The listing builds one solid part. Answer for the finished solid, in the listing's coordinates (mm). Face numbers are marked on the shaded views. Round coordinates to 2 decimals unless told otherwise and drop trailing zeros. Write each loop counter-clockwise with the first axis right and the second up, starting at its lowest first coordinate (ties: lowest second). Pieces come first, ordered by that corner, then holes. Notation, with made-up numbers: (64, 58.5) -> (123, 58.5) arc R5 cw to (123, 65.5) -> close; hole circle Ø11 at (25, 26). An arc over 180 degrees is marked (long way). Write each question's results on one line, items separated by ' | '. Start each with the question number.
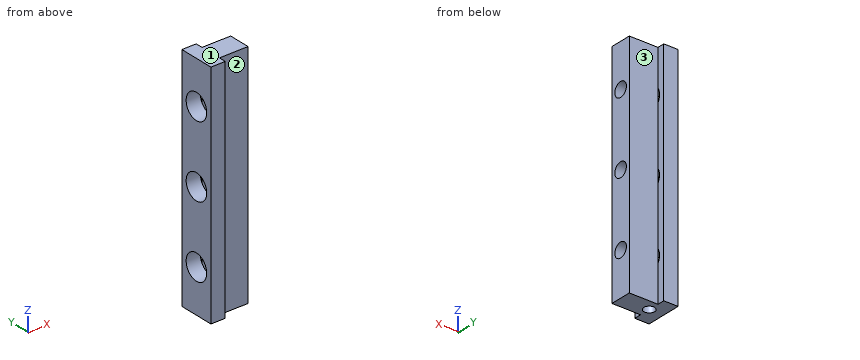
```python
from build123d import *

# Parameters (mm, degrees)
F1_DEPTH = 50.8
F2_R     = 3.175
F3_DEPTH = 19.051
F4_R     = 5.625
F5_DEPTH = 6.4
F6_R     = 2.413
F7_DEPTH = 12.7


with BuildPart() as f1:
    # F0 (on Top) → F1 (new body, symmetric)
    with BuildSketch(Plane.XY):
        Polygon((6.35, 7.9375), (0, 7.9375), (0, -7.9375), (6.35, -7.9375), (6.35, -4.7625), (16.637, -4.7625), (19.05, -4.7625), (19.05, 4.7625), (16.637, 4.7625), (6.35, 4.7625), align=None)
    extrude(amount=F1_DEPTH, both=True)

    # F2 (on face) → F3 (cut, through all)
    with BuildSketch(Plane(origin=(0, 0, 0), x_dir=(0, -1, 0), z_dir=(-1, 0, 0))):
        with Locations((0, 31.75)):
            Circle(F2_R)
        Circle(F2_R)
        with Locations((0, -31.75)):
            Circle(F2_R)
    extrude(amount=-F3_DEPTH, mode=Mode.SUBTRACT)

    # F4 (on face) → F5 (cut)
    with BuildSketch(Plane(origin=(0, 0, 0), x_dir=(0, -1, 0), z_dir=(-1, 0, 0))):
        with Locations((0, 31.75)):
            Circle(F4_R)
        Circle(F4_R)
        with Locations((0, -31.75)):
            Circle(F4_R)
    extrude(amount=-F5_DEPTH, mode=Mode.SUBTRACT)

    # F6 (on face) → F7 (cut)
    with BuildSketch(Plane(origin=(0, 0, -50.8), x_dir=(1, 0, 0), z_dir=(0, 0, -1))):
        with Locations((6.35, 0)):
            Circle(F6_R)
    extrude(amount=-F7_DEPTH, mode=Mode.SUBTRACT)


solid = f1.part
```
Q1. Determine the mould class of the marked faces 1, 2 and 3 for opening direction Y: pulls with the +Y half, pulls with the -Y half, needs draft (parallel to the pull), parting line crosses it, or undercut.
Q2. The part is cut by section D-D, the plane z = 27.5. Write down the section's boundary in (x, y).
Q3. The part is cut by section A-A, the plane z = 0. State how many separate pieces and enclosed holes the cut face has, then the cut area to 3 significant figures.
Q4. Each of these flat-tipped pins is pushed along its axis until it touches: pin 1 (7.5 mm diameter, centred on y = 0, z = 32, fed in from -X); pin 2 (4 mm diameter, centred on x = 6.35, y = 0, fed in from -Z); pin 3 (2 mm diameter, centred on y = 3, z = -7, fed in from -X); pin 4 (5 mm diameter, centred on x = 9, z = 33.5, fed in from -Y). Where does it stop, or does it pass through?
Q5. Find the intervals of material crossed by line 1 (Z direction, x = 2.25, y = 0) (3 decimals); line 2 (Z direction, x = 5, y = 0) (3 decimals); line 3 (X direction, y = 0, z = -46.5), in increasing order.
Answers follow:
1) face 1: needs draft | face 2: pulls with the -Y half | face 3: pulls with the +Y half
2) outline: (0, -7.94) -> (6.35, -7.94) -> (6.35, -4.76) -> (19.05, -4.76) -> (19.05, 4.76) -> (6.35, 4.76) -> (6.35, 7.94) -> (0, 7.94) -> (0, 3.68) -> (6.4, 3.68) -> (6.4, -3.68) -> (0, -3.68) -> close
3) separate pieces: 4 | enclosed holes: 0 | area: 69.5 mm^2
4) pin 1: x = 6.4 | pin 2: z = -38.1 | pin 3: x = 0 | pin 4: y = -4.76
5) line 1: -50.8 to -37.375, -26.125 to -5.625, 5.625 to 26.125, 37.375 to 50.8 | line 2: -38.1 to -37.375, -26.125 to -5.625, 5.625 to 26.125, 37.375 to 50.8 | line 3: 0 to 3.94, 8.76 to 19.05
